Read the model definition and answer for the solid it produces. Units are mm, in the model's axes. A direction names the side the tool comes from. Coordinates: 2 decimals unless noted, no trailing zeros. Loops run counter-clockwise (first coordinate to the right, second up) from the corner with the lowest first, then second, coordinate; pieces in that order, holes last.
Q1. Flat-ended cylindrical pins translate along their axes: P1, Ø10, axis at x = -13.5, z = 5.5, coming from the -Y side; P2, Ø4, axis at x = -3, z = -1, coming from the -Y side; P3, Ø0.8, axis at y = 5, z = 11, coming from the -X side. Find the tip coordinate at first contact, or state that the pin passes through.
Q2. Section A-A (z = 4) is taken. Give the vertices of the cut face in (x, y).
Q3. Straight lines are drawn through the part: line 1 (Z direction, x = -8, y = -2); line 2 (Y direction, x = 10, z = -4.5); line 3 (Y direction, x = -8, z = -0.5). For each, find the intervals that lie inside material, in ascending order.
Q4. Section C-C (z = -4.5) is taken. Give the vertices of the cut face in (x, y).
Q5. Section B-B (z = -1.5) is taken. Give the vertices of the cut face in (x, y), then the cut area to 3 significant figures.
Q6. The mould has two halves that part along X. Classify faces 1 (the face through (10.793, -6.859, 11.448)), 2 (the face through (16.509, 1, -4)), 3 (the face through (-10.246, -13.237, 12.318)), 4 (the face through (0, 1.27, -2)): pulls with the +X half, pulls with the -X half, needs draft (parallel to the pull), parting line crosses it, or undercut.
Q7. Which of the six approach directions +Z, -Z, +X, -X, +Y, -Y give full straight-line access (tool end or side, diameter ignored) to faces 5 (the face through (-4.477, 3.668, 11.448)), 6 (the face through (4, 1, 12.7))?
from build123d import *

# Parameters (mm, degrees)
F1_DEPTH  = 12.7
F2_R      = 1.27
F3_W      = 33.0184467606
F3_H      = 7.62
F4_DEPTH  = 6.35
F6_DEPTH  = 5.08
F7_R      = 2.54
F8_R      = 1.26999
F10_R     = 0.5243142603
F10_R_2   = 0.598941464
F10_R_3   = 1.9572905624
F10_R_4   = 0.79146579
F11_DEPTH = 2.54


# Not quite as in the source:
# - a fillet or chamfer is up to 0.001 mm smaller than in the source, because OpenCascade refuses the exact size
# - a feature of the source that left no trace in its solid (it failed there, or was rolled back) is left out


with BuildPart() as f1:
    # F0 (on Top) → F1 (new body)
    with BuildSketch(Plane.XY):
        Polygon((0, -27.94), (0, 0), (-20.32, 0), align=None)
        with BuildLine():
            Line((-20.32, 0), (0, 0))
            Line((0, 0), (-13.111957335, 18.7258157324))
            ThreePointArc((-13.111957335, 18.7258157324), (-21.7665907667, 11.3070168981), (-20.32, 0))
        make_face()
        with BuildLine():
            Line((0, 0), (0, 12.7))
            ThreePointArc((0, 12.7), (-5.5495799526, 17.902795111), (-13.111957335, 18.7258157324))
            Line((-13.111957335, 18.7258157324), (0, 0))
        make_face()
        with BuildLine():
            ThreePointArc((13.111957335, 18.7258157324), (5.5495799526, 17.902795111), (0, 12.7))
            Line((0, 12.7), (0, 0))
            Line((0, 0), (13.111957335, 18.7258157324))
        make_face()
        with BuildLine():
            Line((13.111957335, 18.7258157324), (0, 0))
            Line((0, 0), (20.32, 0))
            ThreePointArc((20.32, 0), (21.7665907667, 11.3070168981), (13.111957335, 18.7258157324))
        make_face()
        Polygon((20.32, 0), (0, 0), (0, -27.94), align=None)
    extrude(amount=F1_DEPTH)

    # F2
    f2_edges = [f1.edges().sort_by_distance(p)[0] for p in [
        (0, -27.94, 6.35),
    ]]
    fillet(f2_edges, radius=F2_R)

    # F3 (on face) → F4 (join)
    with BuildSketch(Plane(origin=(0, 0, 0), x_dir=(1, 0, 0), z_dir=(0, 0, -1))):
        Rectangle(F3_W, F3_H)
    extrude(amount=F4_DEPTH)

    # F5 (on face) → F6 (cut)
    with BuildSketch(Plane.XZ.offset(3.81)):
        Polygon((-16.5092233803, -3.81), (0, -3.81), (16.5092233803, -3.81), (16.5092233803, 0), (-16.5092233803, 0), align=None)
    extrude(amount=-F6_DEPTH, mode=Mode.SUBTRACT)

    # F7
    f7_edges = [f1.edges().sort_by_distance(p)[0] for p in [
        (0, 3.81, -6.35),
    ]]
    fillet(f7_edges, radius=F7_R)

    # F8 (radius 1.27 in the source; OpenCascade refuses exactly that, so slightly less here)
    f8_edges = [f1.edges().sort_by_distance(p)[0] for p in [
        (0, -3.81, -3.81),
        (0, -3.81, -6.35),
        (-10.673547, -13.263872, 12.7),
        (10.673547, -13.263872, 0),
    ]]
    fillet(f8_edges, radius=F8_R)

    # F10 (on face) → F11 (cut)
    with BuildSketch(Plane.XY.offset(12.7)):
        Polygon((-7.3335906491, 6.9943653395), (-10.5627283372, 6.9943653395), (-10.5627283372, 0), (-7.3335906491, 0.7349486114), (-7.79060311, 2.7429205143), (-9.3015888706, 3.7297289819), (-9.3015888706, 4.4142501429), (-7.79060311, 5.1843370311), align=None)
        with Locations((-9.2159248888, 1.6810059315)):
            Circle(F10_R, mode=Mode.SUBTRACT)
        with Locations((-9.0948464349, 5.7926201262)):
            Circle(F10_R_2, mode=Mode.SUBTRACT)
        Polygon((-5.2438098937, -3.1229529995), (-7.5429510325, -7.2372052819), (-7.1194251068, -8.2657681778), (-5.6228582704, -6.0908141027), (-4.3273653508, -7.5203236143), (-2.2791281808, -5.6641087867), (-0.5245208158, -7.6002273709), (-1.4925802825, -3.1229529995), (-4.0337359533, -5.60360495), align=None)
        Polygon((-2.0902381511, 3.4230099991), (0, 3.3229410183), (-0.7406336372, 5.1936786622), (-4.1223512962, 5.1936786622), (-4.841865506, 2.0997666288), (-2.8991762083, 0), (0, 0), (0, 1.4977937099), (-2.3469333537, 1.4977937099), (-3.6731935106, 2.6101409458), (-2.9886723496, 4.2358790524), (-1.1918039527, 4.2358790524), align=None)
        Polygon((7.5416904874, 5.4201777093), (6.0734692961, 5.7895942591), (2.8356553521, 4.4944682159), (2.8356553521, 2.7429205143), (6.001518108, 2.0997666288), (6.001518108, 1.4977937099), (2.6644766331, 0), (3.9051719941, 0), (7.2849951684, 1.4977937099), (7.2849951684, 2.6820923667), (4.5469105244, 3.281048499), (4.5469105244, 4.2650480755), align=None)
        Polygon((12.8831379116, 3.8117669891), (11.4310486242, 3.702860409), (11.4310486242, 0), (12.8831379116, 0.5112900399), align=None)
        Polygon((11.4310486242, 3.702860409), (11.4310486242, 4.6575730793), (9.4949305058, 4.2020159308), (8.4058633074, 3.4759717528), align=None)
        Polygon((12.8831379116, 7.8927418217), (11.4310486242, 7.6507278718), (11.4310486242, 4.6575730793), (12.8831379116, 4.999241105), align=None)
        Polygon((15.6663097441, 5.6541049853), (12.8831379116, 4.999241105), (12.8831379116, 3.8117669891), (15.6663097441, 4.0205046535), align=None)
        Polygon((12.8831379116, 4.999241105), (11.4310486242, 4.6575730793), (11.4310486242, 3.702860409), (12.8831379116, 3.8117669891), align=None)
        Polygon((6.9560511038, -5.2067907527), (6.0911364853, -7.59802619), (5.8446256444, -8.1831160933), (6.6077862866, -8.1831160933), (7.0911212824, -6.5296017565), (7.3963850737, -6.5296017565), (7.727087941, -7.801536005), (8.9402683079, -8.0050453544), (9.7322071764, -6.8857432343), (9.7322071764, -8.4376684573), (10.517465882, -8.5646957159), (11.0771171749, -5.1050363109), (9.7034284845, -5.7155638933), (8.9911455289, -6.8348660134), (8.0683877672, -6.8348660134), (8.0683877672, -5.6091251385), align=None)
        with Locations((3.0384953134, -5.5120550096)):
            Circle(F10_R_3)
        with Locations((3.0384953134, -5.5120550096)):
            Circle(F10_R_4, mode=Mode.SUBTRACT)
    extrude(amount=-F11_DEPTH, mode=Mode.SUBTRACT)


solid = f1.part
Numbers:
1. P1: stops at y = -16.25
1. P2: stops at y = -25.2
1. P3: stops at x = -22.46
2. outline: (-20.32, 0) - (-1.03, -26.53) arc R1.27 ccw to (1.03, -26.53) - (20.32, 0) arc R12.01 ccw (long way) to (0, 12.7) arc R12.01 ccw (long way) to start
3. line 1: z = -6.35 to -3.81, 0 to 12.7
3. line 2: y = -3.67 to 3.71
3. line 3: y = 1.27 to 3.81
4. outline: (-16.51, -3.67) - (16.51, -3.67) - (16.51, 3.71) - (-16.51, 3.71) - close
5. outline: (-16.51, 1.27) - (16.51, 1.27) - (16.51, 3.81) - (-16.51, 3.81) - close
5. area: 83.9 mm2
6. face 1: undercut
6. face 2: pulls with the +X half
6. face 3: pulls with the -X half
6. face 4: needs draft
7. face 5: +Z
7. face 6: +Z, +X, -X, +Y, -Y
